Verification items for this drawing (mm, ordinates from the low corner). Coordinates: 2 decimals unless noted, no trailing zeros. Order: outer loops, then holes, each group sorted by start corner. A loop starts at its lowest first (then second) coordinate and runs counter-clockwise, first axis right, second up.
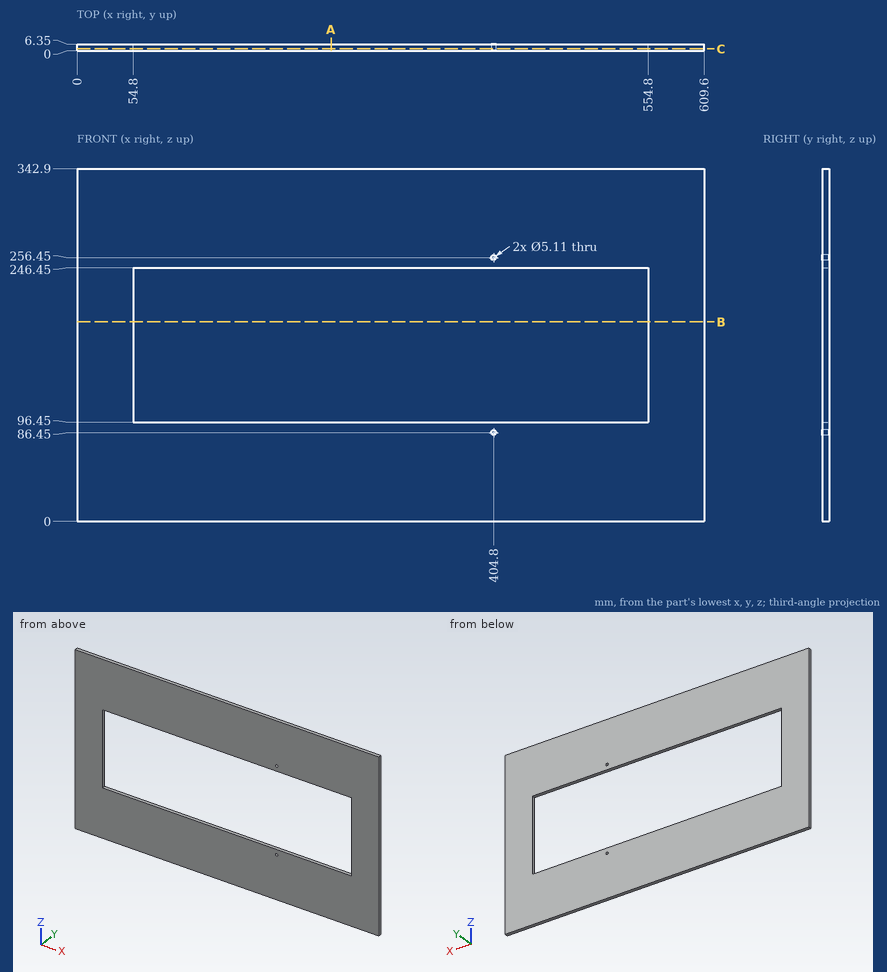
(1) Cross-section at B-B (z = 194). Enter the section's corners in (x, y).
Filled in:
outline: (0, 0) - (54.8, 0) - (54.8, 6.35) - (0, 6.35) - close; (554.8, 0) - (609.6, 0) - (609.6, 6.35) - (554.8, 6.35) - close
(2) Cross-section at C-C (y = 1.5). Enter the section's corners in (x, z) (3 decimals), and give its area (3 significant figures).
Filled in:
outline: (0, 0) - (609.6, 0) - (609.6, 342.9) - (0, 342.9) - close; hole (54.8, 96.45) - (554.8, 96.45) - (554.8, 246.45) - (54.8, 246.45) - close; hole circle Ø5.11 at (404.8, 86.45); hole circle Ø5.11 at (404.8, 256.45)
area: 134,000 mm2
(3) Go/stop test with a flat-tipped pin: P1, Ø6, axis at x = 404.8, z = 256.45, coming from the -Y side. Record where the tip stops, or that it passes through.
Filled in:
P1: stops at y = 0
(4) Cross-section at A-A (x = 247). Enter the section's corners in (y, z), and give its area (3 significant figures).
Filled in:
outline: (0, 0) - (6.35, 0) - (6.35, 96.45) - (0, 96.45) - close; (0, 246.45) - (6.35, 246.45) - (6.35, 342.9) - (0, 342.9) - close
area: 1,220 mm2
(5) Thickness scan on probe 1 along Z at (x, y) = (404.8, 4.25) (3 decimals); probe 2 along X at (y, z) = (4.5, 256.45) (3 decimals); probe 3 along Z at (x, y) = (93.5, 3). Record the ranges inside material, lowest first.
Filled in:
probe 1: z = 0 to 83.895, 89.005 to 96.45, 246.45 to 253.895, 259.005 to 342.9
probe 2: x = 0 to 402.245, 407.355 to 609.6
probe 3: z = 0 to 96.45, 246.45 to 342.9
